Can you work these out from the drawing? Everything is in mm from the part's minimum corner. A direction names the side the tool comes from. Round coordinates to 2 decimals unless told otherwise and drop trailing zeros. Loops run counter-clockwise (first coordinate to the right, second up) from the corner with the lowest first, then second, coordinate; pieces in that order, holes last. Notation, with made-up numbers: M -25,52.25 L 14,52.25 A35 cw 14,85.25 Z; hole C 22,-21.5 d6. An arc over 180 degrees is marked long. Use a Markdown table: item, result.
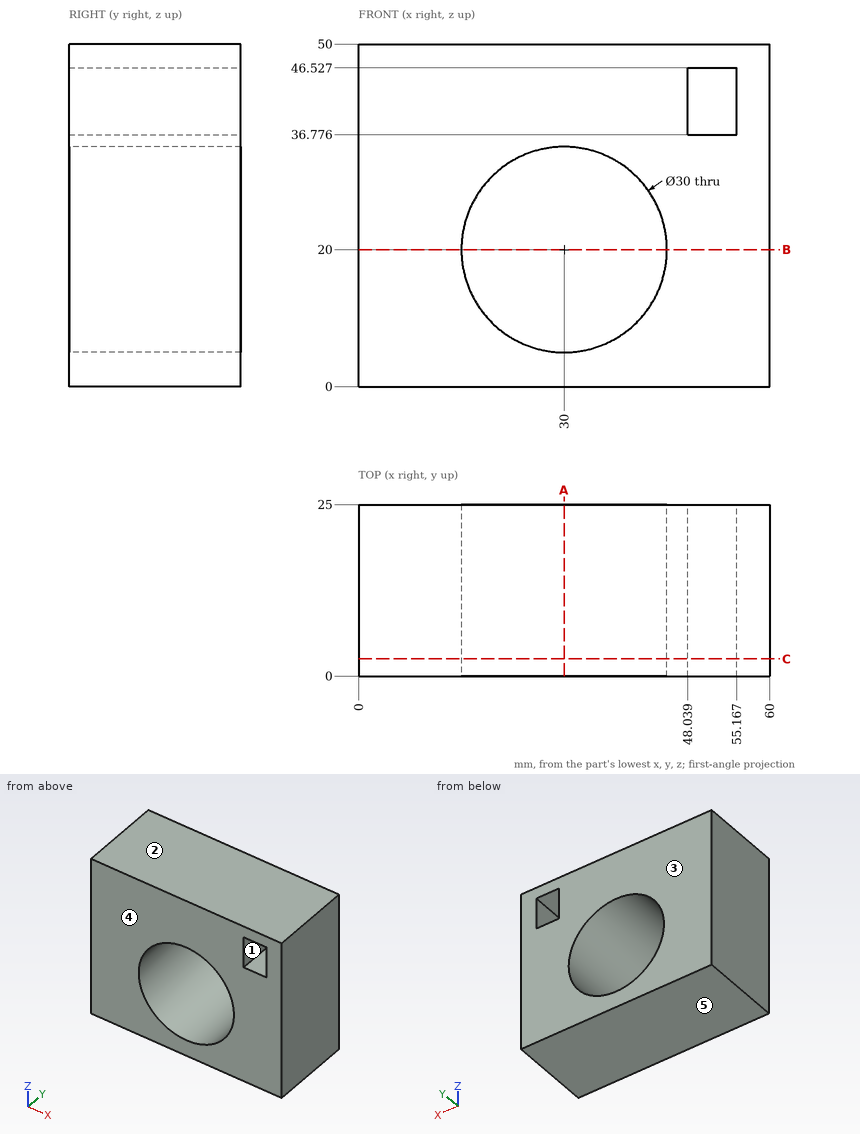
1. I need wall thicknesses on probe 1 along Z at (x, y) = (30, 8); probe 2 along X at (y, z) = (17.5, 45.5); probe 3 along Z at (x, y) = (52.5, 18.5). Which ranges of each line are inside material? Lowest first, please. Write a range as from..to.
Answer sheet:
| item | result |
|---|---|
| probe 1 | 0..5, 35..50 |
| probe 2 | 0..48.04, 55.17..60 |
| probe 3 | 0..36.78, 46.53..50 |
2. We'd pull the mould along Y, two halves only. Please class the marked faces 3, 4 and 5: +Y half, -Y half, draft (parallel to the pull), parting line (faces both ways), or undercut.
Answer sheet:
| item | result |
|---|---|
| face 3 | +Y half |
| face 4 | -Y half |
| face 5 | draft |
3. Imagine slicing it at C-C, the plane y = 2.5. Write out the boundary of the cut face in (x, z), then the cut area to 3 significant figures.
Answer sheet:
| item | result |
|---|---|
| outline | M 0,0 L 60,0 L 60,50 L 0,50 Z; hole C 30,20 d30; hole M 48.04,36.78 L 55.17,36.78 L 55.17,46.53 L 48.04,46.53 Z |
| area | 2,220 mm2 |
4. For pin 1 Ø3.5 at (x, y) = (52, 11) entering from -Z, with a flat end and sliding along its axis, tell me the tip position at first contact or that it passes through.
Answer sheet:
| item | result |
|---|---|
| pin 1 | z = 0 |
5. Which directions (+Z, -Z, +X, -X, +Y, -Y) give clear straight access to the entire face, cutting with the end or side of a thin tool? Please do the marked faces 1 and 2.
Answer sheet:
| item | result |
|---|---|
| face 1 | +Y, -Y |
| face 2 | +Z, +X, -X, +Y, -Y |
6. Imagine slicing it at B-B, the plane z = 20. Write out the boundary of the cut face in (x, y), then the cut area to 3 significant figures.
Answer sheet:
| item | result |
|---|---|
| outline | M 0,0 L 15,0 L 15,25 L 0,25 Z; M 45,0 L 60,0 L 60,25 L 45,25 Z |
| area | 750 mm2 |
7. Imagine slicing it at A-A, the plane x = 30. Write out the boundary of the cut face in (y, z), then the cut area to 3 significant figures.
Answer sheet:
| item | result |
|---|---|
| outline | M 0,0 L 25,0 L 25,5 L 0,5 Z; M 0,35 L 25,35 L 25,50 L 0,50 Z |
| area | 500 mm2 |
